Part model, mm, in its own coordinate system. Round coordinates to 2 decimals unless told otherwise and drop trailing zeros. Loops run counter-clockwise (first coordinate to the right, second up) from the corner with the lowest first, then second, coordinate; pieces in that order, holes last. Notation, with made-up numbers: M 45.5,44 L 57.5,44 A15 cw 57.5,71 Z; hole C 1,-8.75 d9. An arc over 180 degrees is marked long. Put each result on its own line as item: value. Start each with the question number.
```python
from build123d import *

# Parameters (mm, degrees)
F0_W     = 184.15
F0_H     = 254
F1_DEPTH = 3.175
F2_W     = 3.175
F2_H     = 250.825
F2_H_2   = 3.175
F3_DEPTH = 1.5875
F2_W_2   = 6.35
F2_W_3   = 22.225
F2_W_4   = 28.575
F2_W_5   = 34.925
F4_DEPTH = 1.5875


with BuildPart() as f1:
    # F0 (on Top) → F1 (new body)
    with BuildSketch(Plane.XY):
        with Locations((92.075, 127)):
            Rectangle(F0_W, F0_H)
    extrude(amount=F1_DEPTH)

    # F2 (on face) → F3 (cut)
    with BuildSketch(Plane.XY.offset(3.175)):
        with Locations((7.9375, 125.4125)):
            Rectangle(F2_W, F2_H)
        with Locations((33.3375, 125.4125)):
            Rectangle(F2_W, F2_H)
        with Locations((58.7375, 125.4125)):
            Rectangle(F2_W, F2_H)
        with Locations((84.1375, 125.4125)):
            Rectangle(F2_W, F2_H)
        with Locations((115.8875, 252.4125)):
            Rectangle(F2_W, F2_H_2)
        with Locations((147.6375, 252.4125)):
            Rectangle(F2_W, F2_H_2)
        with Locations((115.8875, 125.4125)):
            Rectangle(F2_W, F2_H)
        with Locations((147.6375, 125.4125)):
            Rectangle(F2_W, F2_H)
        with Locations((84.1375, 252.4125)):
            Rectangle(F2_W, F2_H_2)
        with Locations((58.7375, 252.4125)):
            Rectangle(F2_W, F2_H_2)
        with Locations((33.3375, 252.4125)):
            Rectangle(F2_W, F2_H_2)
        with Locations((7.9375, 252.4125)):
            Rectangle(F2_W, F2_H_2)
    extrude(amount=-F3_DEPTH, mode=Mode.SUBTRACT)

    # F2 (on face) → F4 (cut)
    with BuildSketch(Plane.XY.offset(3.175)):
        with Locations((3.175, 252.4125)):
            Rectangle(F2_W_2, F2_H_2)
        with Locations((20.6375, 252.4125)):
            Rectangle(F2_W_3, F2_H_2)
        with Locations((33.3375, 252.4125)):
            Rectangle(F2_W, F2_H_2)
        with Locations((46.0375, 252.4125)):
            Rectangle(F2_W_3, F2_H_2)
        with Locations((7.9375, 252.4125)):
            Rectangle(F2_W, F2_H_2)
        with Locations((58.7375, 252.4125)):
            Rectangle(F2_W, F2_H_2)
        with Locations((71.4375, 252.4125)):
            Rectangle(F2_W_3, F2_H_2)
        with Locations((100.0125, 252.4125)):
            Rectangle(F2_W_4, F2_H_2)
        with Locations((84.1375, 252.4125)):
            Rectangle(F2_W, F2_H_2)
        with Locations((115.8875, 252.4125)):
            Rectangle(F2_W, F2_H_2)
        with Locations((131.7625, 252.4125)):
            Rectangle(F2_W_4, F2_H_2)
        with Locations((147.6375, 252.4125)):
            Rectangle(F2_W, F2_H_2)
        with Locations((166.6875, 252.4125)):
            Rectangle(F2_W_5, F2_H_2)
    extrude(amount=-F4_DEPTH, mode=Mode.SUBTRACT)


solid = f1.part
```
1. Drop a flat-ended pin along its axis: pin 1 (0.8 mm diameter, centred on x = 134, z = 2.5, fed in from +Y) (3 decimals). Give the stop position or say it passes through.
2. Mould opens along X. For faces 1 (the flat face through (85, 128, 1.588)), 2 (the flat face through (46, 127, 3.175)) say: released by +X, released by -X, zero draft, split by the parting line, or undercut.
3. Wall check: L1, parallel to Y at x = 11.5, z = 2.8 (3 decimals). Give the ranges that are in metal, low to high.
4. Cut at A-A, the plane z = 2.2. Give the cut face in (x, y) (3 decimals), and give its area (3 significant figures).
Results list:
1. pin 1: stops at y = 250.825
2. face 1: undercut
2. face 2: zero draft
3. L1: y = 0 to 250.825
4. outline: M 0,0 L 6.35,0 L 6.35,250.825 L 0,250.825 Z; M 9.525,0 L 31.75,0 L 31.75,250.825 L 9.525,250.825 Z; M 34.925,0 L 57.15,0 L 57.15,250.825 L 34.925,250.825 Z; M 60.325,0 L 82.55,0 L 82.55,250.825 L 60.325,250.825 Z; M 85.725,0 L 114.3,0 L 114.3,250.825 L 85.725,250.825 Z; M 117.475,0 L 146.05,0 L 146.05,250.825 L 117.475,250.825 Z; M 149.225,0 L 184.15,0 L 184.15,250.825 L 149.225,250.825 Z
4. area: 41,400 mm^2
